The listing builds one solid part. Answer for the finished solid, in the listing's coordinates (mm). A direction names the side the tool comes from. Give positions to 0.01 mm unless a question says otherwise; leave off trailing zeros. Order: outer loops, then holes, each group sorted by start corner. A loop starts at its lowest first (then second) coordinate and runs counter-clockwise, first axis right, second up. Notation, with made-up numbers: (-25.5, 44) - (-12.5, 44) arc R15 ccw to (-12.5, 72) - close; hole circle Ø8 at (-15, -9). An arc over 180 degrees is marked (long way). Use a Markdown table: item, result. Add a question column.
1) Straight lines are drawn through the part: line 1 (X direction, y = 11.4, z = 67.5); line 2 (X direction, y = -8.55, z = 32.5); line 3 (X direction, y = -9, z = 51.5). For each, find the intervals that lie inside material, in ascending order.
2) Flat-ended cylindrical pins translate along their axes: pin 1 (3 mm diameter, centred on x = 13.5, z = 32.5, fed in from -Y); pin 2 (7.5 mm diameter, centred on x = 4.5, y = -3.5, fed in from +Z); pin 3 (9.5 mm diameter, centred on x = 13.5, z = 7.5, fed in from +Y). Find the tip coordinate at first contact, or state that the pin passes through.
3) Find section A-A, the plane z = 52. Determine the outline of the cut face in (x, y).
4) Find section B-B, the plane y = 3.25. State how many separate pieces and enclosed holes the cut face has, plus the area to 3 significant figures.
5) For faces 1 (the face through (-21.078, 11.251, 66.345)), 2 (the face through (-12, 5, 19.5)), 3 (the face through (18, 10.036, 68)), determine the directions among +Z, -Z, +X, -X, +Y, -Y from which every point of the face is accessible in a straight line to the end or side of a thin tool.
6) The mould has two halves that part along Z. Classify faces 4 (the face through (20, -9.5, 31)), 5 (the face through (18, 8, 65)), 6 (the face through (-25, 0, 39)): released by +Z, released by -Z, zero draft, split by the parting line, or undercut.
7) Find section D-D, the plane x = -9. Determine the outline of the cut face in (y, z), plus the area to 4 significant figures.
8) Find section C-C, the plane z = 13. Determine the outline of the cut face in (x, y).
from build123d import *

# Parameters (mm, degrees)
SKETCH_1_W               = 50
SKETCH_1_H               = 25
EXTRUDE_1_DEPTH          = 70
SKETCH_2_W               = 22
SKETCH_2_H               = 25
CUT_EXTRUDE_1_DEPTH      = 40
SKETCH_3_R               = 4.5
CUT_EXTRUDE_2_DEPTH      = 50
SKETCH_4_R               = 6.5
CUT_EXTRUDE_4_DEPTH      = 5
SKETCH_5_R               = 3
CUT_EXTRUDE_5_DEPTH      = 29
CUT_EXTRUDE_6_DEPTH      = 5
CUT_EXTRUDE_6_DEPTH_BACK = 15
SKETCH_7_W               = 5
SKETCH_7_H               = 15
CUT_EXTRUDE_7_DEPTH      = 10
CUT_EXTRUDE_START        = -10
SKETCH_8_R               = 1.25
CUT_EXTRUDE_8_DEPTH      = 40
SKETCH_9_R               = 2.75
CUT_EXTRUDE_9_DEPTH      = 3
FILLET_2_R               = 5
SKETCH_10_W              = 9
SKETCH_10_H              = 4
CUT_EXTRUDE_10_DEPTH     = 5
SKETCH_12_R              = 1.25
CUT_EXTRUDE_11_DEPTH     = 10


with BuildPart() as part:
    # Sketch 1 → Extrude 1 (new body)
    with BuildSketch(Plane.XY):
        Rectangle(SKETCH_1_W, SKETCH_1_H)
    extrude(amount=EXTRUDE_1_DEPTH)

    # Sketch 2 → Cut-Extrude 1 (cut)
    with BuildSketch(Plane.XY.offset(70)):
        Rectangle(SKETCH_2_W, SKETCH_2_H)
    extrude(amount=-CUT_EXTRUDE_1_DEPTH, mode=Mode.SUBTRACT)

    # Sketch 3 → Cut-Extrude 2 (cut)
    with BuildSketch(Plane(origin=(25, 0, 0), x_dir=(0, 0, -1), z_dir=(1, 0, 0))):
        with Locations((-52, 2.5)):
            Circle(SKETCH_3_R)
    extrude(amount=-CUT_EXTRUDE_2_DEPTH, mode=Mode.SUBTRACT)

    # Sketch 4 → Cut-Extrude 4 (cut)
    with BuildSketch(Plane.ZY.offset(-25)):
        with Locations((52, 2.5)):
            Circle(SKETCH_4_R)
    cut_extrude_4 = extrude(amount=CUT_EXTRUDE_4_DEPTH, mode=Mode.SUBTRACT)

    # Sketch 5 → Cut-Extrude 5 (cut)
    with BuildSketch(Plane(origin=(0, 12.5, 0), x_dir=(1, 0, 0), z_dir=(0, 1, 0))):
        with Locations(Location((16, -9, 0), (0, 0, 270))):
            Circle(SKETCH_5_R)
        with BuildLine():
            Line((16, 12.355747981), (16, 0))
            ThreePointArc((16, 0), (22.363961031, -2.636038969), (25, -9))
            Line((25, -9), (37.355747981, -9))
            ThreePointArc((37.355747981, -9), (31.100794214, 6.100794214), (16, 12.355747981))
        make_face()
    cut_extrude_5 = extrude(amount=-CUT_EXTRUDE_5_DEPTH, mode=Mode.SUBTRACT)

    # Mirror 2: Cut-Extrude 4, Cut-Extrude 5 across plane
    add(cut_extrude_4.mirror(Plane(origin=(0, 0, 0), x_dir=(0, 0, 1), z_dir=(1, 0, 0))), mode=Mode.SUBTRACT)
    add(cut_extrude_5.mirror(Plane(origin=(0, 0, 0), x_dir=(0, 0, 1), z_dir=(1, 0, 0))), mode=Mode.SUBTRACT)

    # Sketch 6 → Cut-Extrude 6 (cut, two sides: drawn at the far end of the back side and taken through both)
    with BuildSketch(Plane(origin=(0, 12.5, 0), x_dir=(1, 0, 0), z_dir=(0, 1, 0)).offset(-CUT_EXTRUDE_6_DEPTH_BACK)):
        Polygon((6, -19.5), (6, 5.258137662), (25, 5.258137662), (25, -14.502176213), (19.043825546, -19.5), align=None)
        Polygon((-25, -14.502176213), (-25, 5.258137662), (-6, 5.258137662), (-6, -19.5), (-19.043825546, -19.5), align=None)
    extrude(amount=CUT_EXTRUDE_6_DEPTH + CUT_EXTRUDE_6_DEPTH_BACK, mode=Mode.SUBTRACT)

    # Sketch 7 → Cut-Extrude 7 (cut)
    with BuildSketch(Plane(origin=(-11, 0, 0), x_dir=(0, 0, -1), z_dir=(1, 0, 0))):
        with Locations((-32.5, 0)):
            Rectangle(SKETCH_7_W, SKETCH_7_H)
    cut_extrude_7 = extrude(amount=-CUT_EXTRUDE_7_DEPTH, mode=Mode.SUBTRACT)

    # Sketch 8 → Cut-Extrude 8 (cut)
    with BuildSketch(Plane(origin=(0, -7.5, 0), x_dir=(1, 0, 0), z_dir=(0, 1, 0)).offset(CUT_EXTRUDE_START)):
        with Locations(Location((-19.574812365, -32.5, 0), (0, 0, 90))):
            Circle(SKETCH_8_R)
        with Locations(Location((-13.5, -32.5, 0), (0, 0, 90))):
            Circle(SKETCH_8_R)
    cut_extrude_8 = extrude(amount=CUT_EXTRUDE_8_DEPTH, mode=Mode.SUBTRACT)

    # Sketch 9 → Cut-Extrude 9 (cut)
    with BuildSketch(Plane.XZ.offset(12.5)):
        with Locations(Location((-19.574812365, 32.5, 0), (0, 0, 270))):
            Circle(SKETCH_9_R)
        with Locations((-13.5, 32.5)):
            Circle(SKETCH_9_R)
    cut_extrude_9 = extrude(amount=-CUT_EXTRUDE_9_DEPTH, mode=Mode.SUBTRACT)

    # Fillet 2
    fillet_2_edges = [part.edges().sort_by_distance(p)[0] for p in [
        (18, -12.5, 70),
        (-18, -12.5, 70),
    ]]
    fillet(fillet_2_edges, radius=FILLET_2_R)

    # Sketch 10 → Cut-Extrude 10 (cut)
    with BuildSketch(Plane.XY.offset(70)):
        with Locations((-18, 8.036191449)):
            Rectangle(SKETCH_10_W, SKETCH_10_H)
    cut_extrude_10 = extrude(amount=-CUT_EXTRUDE_10_DEPTH, mode=Mode.SUBTRACT)

    # Sketch 12 → Cut-Extrude 11 (cut)
    with BuildSketch(Plane.XZ.offset(-10.036191449)):
        with Locations((-15.400835213, 67.5)):
            Circle(SKETCH_12_R)
        with Locations(Location((-20.599164787, 67.5, 0), (0, 0, 270))):
            Circle(SKETCH_12_R)
    cut_extrude_11 = extrude(amount=-CUT_EXTRUDE_11_DEPTH, mode=Mode.SUBTRACT)

    # Mirror 3: Cut-Extrude 7, Cut-Extrude 8, Cut-Extrude 9, Cut-Extrude 10, Cut-Extrude 11 across plane
    add(cut_extrude_7.mirror(Plane(origin=(0, 0, 0), x_dir=(0, 0, 1), z_dir=(1, 0, 0))), mode=Mode.SUBTRACT)
    add(cut_extrude_8.mirror(Plane(origin=(0, 0, 0), x_dir=(0, 0, 1), z_dir=(1, 0, 0))), mode=Mode.SUBTRACT)
    add(cut_extrude_9.mirror(Plane(origin=(0, 0, 0), x_dir=(0, 0, 1), z_dir=(1, 0, 0))), mode=Mode.SUBTRACT)
    add(cut_extrude_10.mirror(Plane(origin=(0, 0, 0), x_dir=(0, 0, 1), z_dir=(1, 0, 0))), mode=Mode.SUBTRACT)
    add(cut_extrude_11.mirror(Plane(origin=(0, 0, 0), x_dir=(0, 0, 1), z_dir=(1, 0, 0))), mode=Mode.SUBTRACT)


solid = part.part
The answers:
| question | item | result |
|---|---|---|
| 1 | line 1 | -25 to -21.85, -19.35 to -16.65, -14.15 to -11, 11 to 14.15, 16.65 to 19.35, 21.85 to 25 |
| 1 | line 2 | -25 to -20.82, -18.32 to -14.75, -12.25 to -11, 11 to 12.25, 14.75 to 18.32, 20.82 to 25 |
| 1 | line 3 | -25 to -11, 11 to 25 |
| 2 | pin 1 | y = -9.5 |
| 2 | pin 2 | z = 30 |
| 2 | pin 3 | y = -2.5 |
| 3 | outline | (-25, -12.5) - (-11, -12.5) - (-11, -2) - (-20, -2) - (-20, -4) - (-25, -4) - close; (-25, 9) - (-20, 9) - (-20, 7) - (-11, 7) - (-11, 12.5) - (-25, 12.5) - close; (11, -12.5) - (25, -12.5) - (25, -4) - (20, -4) - (20, -2) - (11, -2) - close; (11, 7) - (20, 7) - (20, 9) - (25, 9) - (25, 12.5) - (11, 12.5) - close |
| 4 | separate pieces | 3 |
| 4 | enclosed holes | 0 |
| 4 | area | 1,520 mm2 |
| 5 | face 1 | +Y |
| 5 | face 2 | -Z, +Y |
| 5 | face 3 | +Z |
| 6 | face 4 | undercut |
| 6 | face 5 | released by +Z |
| 6 | face 6 | zero draft |
| 7 | outline | (-12.5, 0) - (-2.5, 0) - (-2.5, 19.5) - (12.5, 19.5) - (12.5, 30) - (-12.5, 30) - close |
| 7 | area | 457.5 mm2 |
| 8 | outline | (-25, -12.5) - (25, -12.5) - (25, -2.5) - (6, -2.5) - (6, 12.5) - (-6, 12.5) - (-6, -2.5) - (-25, -2.5) - close |
